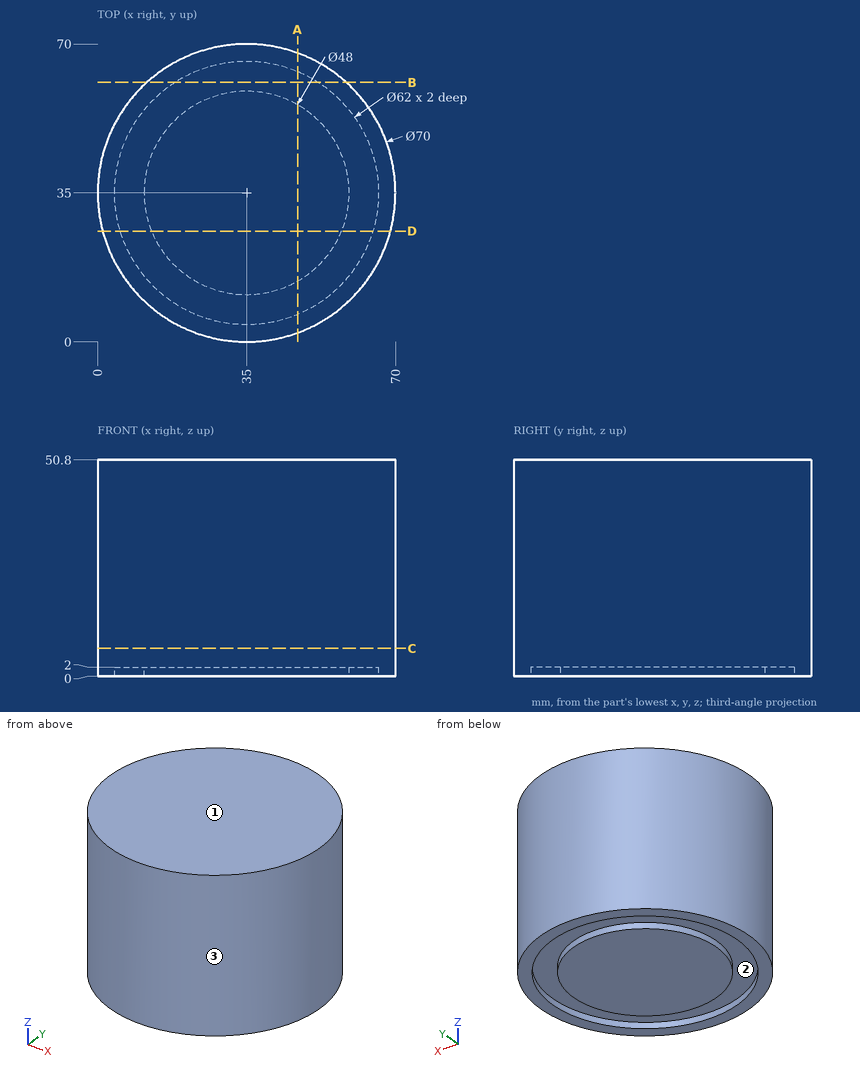
Answer from the drawing. Dimensions are ordinates in mm from the lowest x, y and z of the part. Give positions to 0.01 mm unless a question says otherwise; leave off trailing zeros. Order: outer loops, then holes, each group sorted by start corner. A loop starts at its lowest first (then second) coordinate and runs counter-clockwise, first axis right, second up. Notation, with made-up numbers: (18.25, 25) -> (56.25, 25) arc R23 cw to (56.25, 61) -> close; hole circle Ø1 at (-34, 42). An arc over 180 degrees is marked (long way). Answer as a JSON object with one key per item and string values. Group by question number.
1. Section B-B on y = 61 is taken. Determine the outline of the cut face in (x, z), plus the area to 3 significant figures.
2. Section D-D on y = 26 is taken. Determine the outline of the cut face in (x, z), plus the area to 3 significant figures.
3. Consider line 1 along Y through (x, z) = (35, 0.95); line 2 along Z through (x, y) = (42.5, 58); line 3 along X through (y, z) = (13, 24). Determine where each line is inside the solid, lowest interval first. Write a range as [from, to].
4. The mould has two halves that part along Y. Classify the marked faces 1, 2 and 3: released by +Y, released by -Y, zero draft, split by the parting line, or undercut.
5. Section C-C on z = 6.5 is taken. Determine the outline of the cut face in (x, y), plus the area to 3 significant figures.
6. Flat-ended cylindrical pins translate along their axes: pin 1 Ø6 at (x, z) = (56, 45.5) entering from +Y; pin 2 Ø5 at (y, z) = (61, 6) entering from -X; pin 3 Ø1.5 at (y, z) = (18.5, 34.5) entering from -X. Find the tip coordinate at first contact, or state that the pin passes through.
7. Section A-A on x = 47 is taken. Determine the outline of the cut face in (y, z).
Result sheet:
{
 "1": {"outline": "(11.57, 0) -> (18.12, 0) -> (18.12, 2) -> (51.88, 2) -> (51.88, 0) -> (58.43, 0) -> (58.43, 50.8) -> (11.57, 50.8) -> close", "area": "2,310 mm^2"},
 "2": {"outline": "(1.18, 0) -> (5.34, 0) -> (5.34, 2) -> (12.75, 2) -> (12.75, 0) -> (57.25, 0) -> (57.25, 2) -> (64.66, 2) -> (64.66, 0) -> (68.82, 0) -> (68.82, 50.8) -> (1.18, 50.8) -> close", "area": "3,410 mm^2"},
 "3": {"line 1": "y = [0, 4], [11, 59], [66, 70]", "line 2": "z = [2, 50.8]", "line 3": "x = [7.78, 62.22]"},
 "4": {"face 1": "zero draft", "face 2": "undercut", "face 3": "split by the parting line"},
 "5": {"outline": "circle Ø70 at (35, 35)", "area": "3,850 mm^2"},
 "6": {"pin 1": "stops at y = 65.02", "pin 2": "stops at x = 9.06", "pin 3": "stops at x = 3.74"},
 "7": {"outline": "(2.12, 0) -> (6.42, 0) -> (6.42, 2) -> (14.22, 2) -> (14.22, 0) -> (55.78, 0) -> (55.78, 2) -> (63.58, 2) -> (63.58, 0) -> (67.88, 0) -> (67.88, 50.8) -> (2.12, 50.8) -> close"}
}
